```python
from build123d import *

# Parameters (mm, degrees)
CUT_EXTRUDE2_START = -5.08
SKETCH2_R          = 1.778
CUT_EXTRUDE2_DEPTH = 5.08
SKETCH4_R          = 2.413
CUT_EXTRUDE3_DEPTH = 19.05
FILLET1_R          = 1.524


with BuildPart() as part:
    # Sketch1 → Revolve1 (revolve)
    with BuildSketch(Plane(origin=(0, 0, 0), x_dir=(1, 0, 0), z_dir=(0, 1, 0))):
        Polygon((2.701636364, 33.504909091), (2.701636364, 30.456909091), (-16.348363636, 30.456909091), (-16.348363636, 5.056909091), (-22.698363636, 5.056909091), (-22.698363636, 33.504909091), align=None)
    revolve(axis=Axis((-22.698363636, 0, -5.056909091), (0, 0, -1)))

    # Sketch2 → Cut-Extrude2 (cut)
    with BuildSketch(Plane(origin=(0, 0, -33.504909091), x_dir=(-1, 0, 0), z_dir=(0, 0, -1)).offset(CUT_EXTRUDE2_START)):
        with Locations((22.698363636, -19.05)):
            Circle(SKETCH2_R)
        with Locations((22.698363636, 19.05)):
            Circle(SKETCH2_R)
        with BuildLine():
            Line((41.748363636, -5.08), (47.585179423, -5.08))
            ThreePointArc((47.585179423, -5.08), (48.098363636, 0), (47.585179423, 5.08))
            Line((47.585179423, 5.08), (41.748363636, 5.08))
            ThreePointArc((41.748363636, 5.08), (36.668363636, 0), (41.748363636, -5.08))
        make_face()
        with BuildLine():
            Line((3.648363636, 5.08), (-2.18845215, 5.08))
            ThreePointArc((-2.18845215, 5.08), (-2.701636364, 0), (-2.18845215, -5.08))
            Line((-2.18845215, -5.08), (3.648363636, -5.08))
            ThreePointArc((3.648363636, -5.08), (8.728363636, 0), (3.648363636, 5.08))
        make_face()
    extrude(amount=CUT_EXTRUDE2_DEPTH, mode=Mode.SUBTRACT)

    # Sketch4 → Cut-Extrude3 (cut)
    with BuildSketch(Plane.XY.offset(-5.056909091)):
        with Locations((-22.698363636, 0)):
            Circle(SKETCH4_R)
    extrude(amount=-CUT_EXTRUDE3_DEPTH, mode=Mode.SUBTRACT)

    # Fillet1
    fillet1_edges = [part.edges().sort_by_distance(p)[0] for p in [
        (-47.585179423, 5.08, -31.980909091),
        (-47.585179423, -5.08, -31.980909091),
        (2.18845215, -5.08, -31.980909091),
        (2.18845215, 5.08, -31.980909091),
    ]]
    fillet(fillet1_edges, radius=FILLET1_R)


solid = part.part
```
The listing builds one solid part. Answer for the finished solid, in the listing's coordinates (mm). A direction names the side the tool comes from. Round coordinates to 2 decimals unless told otherwise and drop trailing zeros. Loops run counter-clockwise (first coordinate to the right, second up) from the corner with the lowest first, then second, coordinate; pieces in that order, holes last.
1) A cutting plane is placed at B-B on y = 0. Determine the outline of the cut face in (x, z).
Outcome:
outline: (-36.67, -33.5) - (-8.73, -33.5) - (-8.73, -30.46) - (-16.35, -30.46) - (-16.35, -5.06) - (-20.29, -5.06) - (-20.29, -24.11) - (-25.11, -24.11) - (-25.11, -5.06) - (-29.05, -5.06) - (-29.05, -30.46) - (-36.67, -30.46) - close
2) A cutting plane is placed at A-A on x = -22.5. Determine the outline of the cut face in (y, z), plus the area to 3 significant figures.
Outcome:
outline: (-25.4, -33.5) - (-20.82, -33.5) - (-20.82, -30.46) - (-25.4, -30.46) - close; (-17.28, -33.5) - (17.28, -33.5) - (17.28, -30.46) - (6.35, -30.46) - (6.35, -5.06) - (2.4, -5.06) - (2.4, -24.11) - (-2.4, -24.11) - (-2.4, -5.06) - (-6.35, -5.06) - (-6.35, -30.46) - (-17.28, -30.46) - close; (20.82, -33.5) - (25.4, -33.5) - (25.4, -30.46) - (20.82, -30.46) - close
area: 364 mm2
3) Given P1, Ø1.4, axis at x = -22, y = 0, coming from the +Z side; P2, Ø1.5, axis at x = -2, z = -31.5, coming from the +Y side; P3, Ø6, axis at x = -26, z = -27, coming from the +Y side; P4, Ø14.5, axis at x = -29.5, y = -10.5, coming from the +Z side, each flat-ended and moving along its own axis, determine where each tip first touches the part or whether it passes through.
Outcome:
P1: stops at z = -24.11
P2: stops at y = 15.72
P3: stops at y = 6.34
P4: stops at z = -5.06
4) A cutting plane is placed at D-D on z = -21.25. Determine the outline of the cut face in (x, y), plus the area to 3 significant figures.
Outcome:
outline: circle Ø12.7 at (-22.7, 0); hole circle Ø4.83 at (-22.7, 0)
area: 108 mm2
5) A cutting plane is placed at C-C on y = 19.05. Determine the outline of the cut face in (x, z), plus the area to 3 significant figures.
Outcome:
outline: (-39.5, -33.5) - (-24.48, -33.5) - (-24.48, -30.46) - (-39.5, -30.46) - close; (-20.92, -33.5) - (-5.9, -33.5) - (-5.9, -30.46) - (-20.92, -30.46) - close
area: 91.6 mm2
6) For a pull along Y with two mould halves and no side action, classify faces 5 (the face through (-16.642, -1.907, -17.579)), 6 (the face through (-18, 5, -30.457)), 7 (the face through (1.45, 5.67, -32)) as released by +Y, released by -Y, zero draft, split by the parting line, or undercut.
Outcome:
face 5: split by the parting line
face 6: zero draft
face 7: undercut
7) For faces 1 (the face through (-44, 5.08, -32)), 2 (the face through (-21.287, -20.132, -31.96)), 3 (the face through (-23, 0, -24.107)), 4 (the face through (-2, 5.08, -32)), determine the directions among +Z, -Z, +X, -X, +Y, -Y from which every point of the face is accessible in a straight line to the end or side of a thin tool.
Outcome:
face 1: +Z, -Z, -X
face 2: +Z, -Z
face 3: +Z
face 4: +Z, -Z, +X
8) Consider line 1 (Z direction, x = -24.5, y = -23); line 2 (X direction, y = -19.05, z = -32.3); line 3 (Y direction, x = -21, z = -7.5). Determine where each line is inside the solid, lowest interval first.
Outcome:
line 1: z = -33.5 to -30.46
line 2: x = -39.5 to -24.48, -20.92 to -5.9
line 3: y = -6.12 to -1.71, 1.71 to 6.12
